Here's how the part is built. I have some questions about the finished solid (model axes, mm). Face numbers are marked on the shaded views. Round coordinates to 2 decimals unless told otherwise and drop trailing zeros. Loops run counter-clockwise (first coordinate to the right, second up) from the corner with the lowest first, then second, coordinate; pieces in that order, holes last. Notation, with made-up numbers: M -27,34.5 L 15,34.5 A14 cw 15,42.5 Z; hole C 24.25,20 d8. An arc over 180 degrees is marked long. Use a Markdown table: item, result.
```python
from build123d import *

# Parameters (mm, degrees)
SKETCH1_R               = 60
BOSS_EXTRUDE1_DEPTH     = 4.5
SKETCH2_R               = 29.275
BOSS_EXTRUDE2_DEPTH     = 56.5
CUT_EXTRUDE1_DEPTH      = 105.503588455
CUT_EXTRUDE1_DEPTH_BACK = 105.503588455
SKETCH3_R               = 26.75
SKETCH4_R               = 32.341067561
SKETCH4_R_2             = 29.275
BOSS_EXTRUDE3_DEPTH     = 56.5
CUT_EXTRUDE2_START      = -4.5
SKETCH5_R               = 32.341067561
SKETCH5_R_2             = 29
CUT_EXTRUDE2_DEPTH      = 4.5
CUT_EXTRUDE3_DEPTH      = 105.503588455
CUT_EXTRUDE3_DEPTH_BACK = 105.503588455
SKETCH6_R               = 1.25


with BuildPart() as part:
    # Sketch1 → Boss-Extrude1 (new body)
    with BuildSketch(Plane(origin=(0, 0, 0), x_dir=(1, 0, 0), z_dir=(0, 1, 0))):
        with Locations(Location((0, 0, 0), (0, 0, 270))):
            Circle(SKETCH1_R)
    extrude(amount=BOSS_EXTRUDE1_DEPTH)

    # Sketch2 → Boss-Extrude2 (add)
    with BuildSketch(Plane(origin=(0, 4.5, 0), x_dir=(1, 0, 0), z_dir=(0, 1, 0))):
        with Locations(Location((0, 0, 0), (0, 0, 270))):
            Circle(SKETCH2_R)
    extrude(amount=BOSS_EXTRUDE2_DEPTH)

    # Sketch3 → Cut-Extrude1 (cut, two sides: drawn at the far end of the back side and taken through both)
    with BuildSketch(Plane(origin=(0, 61, 0), x_dir=(1, 0, 0), z_dir=(0, 1, 0)).offset(-CUT_EXTRUDE1_DEPTH_BACK)):
        with Locations(Location((0, 0, 0), (0, 0, 270))):
            Circle(SKETCH3_R)
    extrude(amount=CUT_EXTRUDE1_DEPTH + CUT_EXTRUDE1_DEPTH_BACK, mode=Mode.SUBTRACT)

    # Sketch4 → Boss-Extrude3 (add)
    with BuildSketch(Plane(origin=(0, 4.5, 0), x_dir=(1, 0, 0), z_dir=(0, 1, 0))):
        with Locations(Location((0, 0, 0), (0, 0, 270))):
            Circle(SKETCH4_R)
        Circle(SKETCH4_R_2, mode=Mode.SUBTRACT)
    extrude(amount=BOSS_EXTRUDE3_DEPTH)

    # Sketch5 → Cut-Extrude2 (cut)
    with BuildSketch(Plane(origin=(0, 61, 0), x_dir=(1, 0, 0), z_dir=(0, 1, 0)).offset(CUT_EXTRUDE2_START)):
        with Locations(Location((0, 0, 0), (0, 0, 270))):
            Circle(SKETCH5_R)
        with Locations(Location((0, 0, 0), (0, 0, 270))):
            Circle(SKETCH5_R_2, mode=Mode.SUBTRACT)
    extrude(amount=CUT_EXTRUDE2_DEPTH, mode=Mode.SUBTRACT)

    # Sketch6 → Cut-Extrude3 (cut, two sides: drawn at the far end of the back side and taken through both)
    with BuildSketch(Plane.XZ.offset(-CUT_EXTRUDE3_DEPTH_BACK)):
        with Locations(Location((31.819805153, -31.819805153, 0), (0, 0, 270))):
            Circle(SKETCH6_R)
        with Locations(Location((0, 45, 0), (0, 0, 270))):
            Circle(SKETCH6_R)
        with Locations(Location((31.819805153, 31.819805153, 0), (0, 0, 270))):
            Circle(SKETCH6_R)
        with Locations(Location((45, 0, 0), (0, 0, 270))):
            Circle(SKETCH6_R)
        with Locations(Location((-31.819805153, 31.819805153, 0), (0, 0, 270))):
            Circle(SKETCH6_R)
        with Locations(Location((-45, 0, 0), (0, 0, 270))):
            Circle(SKETCH6_R)
        with Locations(Location((-31.819805153, -31.819805153, 0), (0, 0, 270))):
            Circle(SKETCH6_R)
        with Locations(Location((0, -45, 0), (0, 0, 270))):
            Circle(SKETCH6_R)
    extrude(amount=CUT_EXTRUDE3_DEPTH + CUT_EXTRUDE3_DEPTH_BACK, mode=Mode.SUBTRACT)


solid = part.part
```
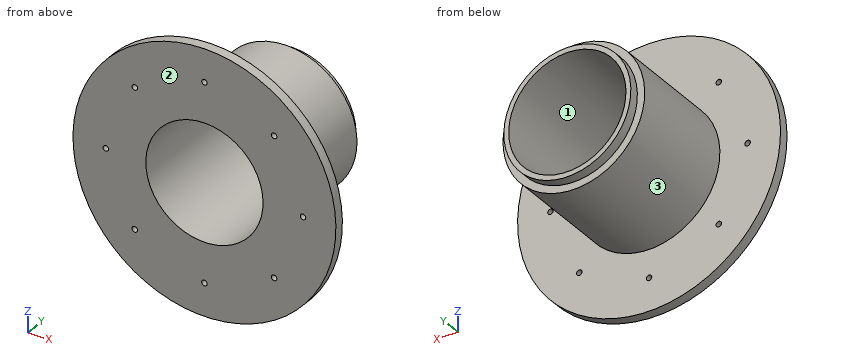
Q1. Imagine slicing it at A-A, the plane z = -7.5. Please give me the cut outline in (x, y).
Return value:
| item | result |
|---|---|
| outline | M -59.53,0 L -25.68,0 L -25.68,61 L -28.01,61 L -28.01,56.5 L -31.46,56.5 L -31.46,4.5 L -59.53,4.5 Z; M 25.68,0 L 59.53,0 L 59.53,4.5 L 31.46,4.5 L 31.46,56.5 L 28.01,56.5 L 28.01,61 L 25.68,61 Z |
Q2. Imagine slicing it at C-C, the plane y = 19. Please give me the cut outline in (x, z).
Return value:
| item | result |
|---|---|
| outline | C 0,0 d64.68; hole C 0,0 d53.5 |
Q3. Imagine slicing it at D-D, the plane x = -39.5. Please give me the cut outline in (y, z).
Return value:
| item | result |
|---|---|
| outline | M 0,-45.16 L 4.5,-45.16 L 4.5,45.16 L 0,45.16 Z |
Q4. I need wall thicknesses on line 1 (X direction, y = 19.5, z = 0); line 2 (Y direction, x = 30, z = -7); line 3 (Y direction, x = -8.5, z = 48.5). Which ranges of each line are inside material? Lowest first, please. Write a range as from..to.
Return value:
| item | result |
|---|---|
| line 1 | x = -32.34..-26.75, 26.75..32.34 |
| line 2 | y = 0..56.5 |
| line 3 | y = 0..4.5 |
Q5. Will these pins go through, and if not, where does the flat tip stop? P1, Ø5, axis at y = 39.5, z = 24, coming from the -X side; P2, Ø3, axis at x = -31.82, z = -31.82, coming from the +Y side; P3, Ø3, axis at y = 24.5, z = 13.5, coming from the +X side.
Return value:
| item | result |
|---|---|
| P1 | stops at x = -24.16 |
| P2 | stops at y = 4.5 |
| P3 | stops at x = 30.03 |
Q6. We'd pull the mould along Z, two halves only. Please class the marked faces 1, 2 and 3: pulls with the +Z half, pulls with the -Z half, needs draft (parallel to the pull), parting line crosses it, or undercut.
Return value:
| item | result |
|---|---|
| face 1 | undercut |
| face 2 | needs draft |
| face 3 | parting line crosses it |
Q7. Imagine slicing it at B-B, the plane x = 21. Please give me the cut outline in (y, z).
Return value:
| item | result |
|---|---|
| outline | M 0,-56.2 L 4.5,-56.2 L 4.5,-24.6 L 56.5,-24.6 L 56.5,-20 L 61,-20 L 61,-16.57 L 0,-16.57 Z; M 0,16.57 L 61,16.57 L 61,20 L 56.5,20 L 56.5,24.6 L 4.5,24.6 L 4.5,56.2 L 0,56.2 Z |
